Autodesk Inventor part; units mm, degrees
ref_plane "YZ Plane" through (0, 0, 0) normal (1, 0, 0) x (0, 1, 0)
ref_plane "XZ Plane" through (0, 0, 0) normal (0, 1, 0) x (-1, 0, 0)
ref_plane "XY Plane" through (0, 0, 0) normal (0, 0, 1) x (1, 0, 0)
sketch "Sketch3" plane through (0, 0, 0) normal (0, 0, 1) x (1, 0, 0)
  circle A0 centre (0, 0) radius 2.5
  dimension "Diameter" = 5
extrude "Extrusion1" add sketch "Sketch3" against normal blind 60
sketch "Sketch4" plane through (0, 0, 0) normal (0, 0, 1) x (1, 0, 0)
  circle A0 centre (0, 0) radius 2.5
  circle A1 centre (0, 0) radius 4.25
  dimension "Head_Diameter" = 8.5
extrude "Extrusion2" add sketch "Sketch4" along normal blind 5 contours A0 | A1
sketch "Sketch5" plane through (0, 0, 5) normal (0, 0, 1) x (1, 0, 0)
  circle A0 centre (0, 0) radius 4.25
  line L0 (2.3094, 0) -> (1.1547, -2)
  line L1 (1.1547, -2) -> (-1.1547, -2)
  line L2 (-1.1547, -2) -> (-2.3094, 0)
  line L3 (-2.3094, 0) -> (-1.1547, 2)
  line L4 (-1.1547, 2) -> (1.1547, 2)
  line L5 (1.1547, 2) -> (2.3094, 0)
  line L6 (0, 0) -> (2.3094, 0) construction
  dimension "Hex_Width" = 4
extrude "Extrusion3" cut sketch "Sketch5" against normal blind 2.5 contours L0 L1 L2 L3 L4 L5
thread "Thread1"
chamfer "Chamfer1" distance 0.5 angle 45 1 edges at (-4.25, 0, 5)
chamfer "Chamfer2" distance 0.25 angle 45 1 edges at (-2.5, 0, -60)
equation "\"d14\" = 0.5 * Chamfer"
properties part number "SCREW,SOCKET HD,P,12.9,M5X0.8X60MM" material "Steel, MS"
Input: part model. Units: mm. Frame: model coordinates. A direction names the side the tool comes from. Coordinates: 2 decimals unless noted, no trailing zeros. Loops run counter-clockwise (first coordinate to the right, second up) from the corner with the lowest first, then second, coordinate; pieces in that order, holes last. Notation, with made-up numbers: (19, 69) -> (49, 69) arc R13 cw to (49, 79) -> close; hole circle Ø2 at (37, 51). An arc over 180 degrees is marked (long way). Write item = value, one per line. Start each with the question number.
Item 1: Mould query, pull axis Y, two halves, no side actions, for faces 1 (the face through (2, -2, 0)), 2 (the face through (1.724, 1.014, 3.768)), 3 (the face through (-0.54, -2.44, -29.46)). Classes: pulls with the +Y half, pulls with the -Y half, needs draft (parallel to the pull), parting line crosses it, or undercut.
Item 2: Material intervals for line 1 (Z direction, x = 2.75, y = 0.75); line 2 (Y direction, x = -1.5, z = -4.5); line 3 (Y direction, x = 0, z = -40), sorted ascending.
Item 3: Cut plane A-A, the plane x = 0. Return loops of the section in (y, z).
Item 4: Reachability of faces 4 (the face through (0, -2, 4)), 5 (the face through (2.285, -3.584, 2.218)) from +Z, -Z, +X, -X, +Y, -Y: full face, straight path, thin tool, end or side. Return the list, or none.
Item 5: First-contact query: P1, Ø4, axis at y = -2, z = -22.5, coming from the -X side; P2, Ø2, axis at x = 1.5, z = -27, coming from the -Y side; P3, Ø1.5, axis at y = 2, z = -33, coming from the -X side. Flat tips, straight axial feed; report the tip coordinate or a pass-through.
Item 6: Cut plane B-B, the plane z = -5. Return loops of the section in (x, y), plus the area to 3 significant figures.
Ans:
q1.face_1 = needs draft
q1.face_2 = undercut
q1.face_3 = parting line crosses it
q2.line_1 = 0 to 5
q2.line_2 = -2 to 2
q2.line_3 = -2.5 to 2.5
q3.outline = (-4.25, 0) -> (-2.5, 0) -> (-2.5, -59.75) -> (-2.25, -60) -> (2.25, -60) -> (2.5, -59.75) -> (2.5, 0) -> (4.25, 0) -> (4.25, 4.5) -> (3.75, 5) -> (2, 5) -> (2, 2.5) -> (-2, 2.5) -> (-2, 5) -> (-3.75, 5) -> (-4.25, 4.5) -> close
q4.face_4 = +Z
q4.face_5 = +Z, -Z
q5.P1 = -2.5
q5.P2 = -2.45
q5.P3 = -2.17
q6.outline = circle Ø5 at (0, 0)
q6.area = 19.6 mm²
